Geometry: final body of the model. Coordinates: model frame, mm. A direction names the side the tool comes from. Coordinates: 2 decimals unless noted, no trailing zeros. Order: outer loops, then holes, each group sorted by start corner. A loop starts at its lowest first (then second) coordinate and runs counter-clockwise, first axis right, second up. Notation, with made-up numbers: M -17,70 L 40,70 A26 ccw 40,106 Z; hole C 59,-6.75 d6. An arc over 180 degrees is marked long. Write item = value, one per line.
from build123d import *

# Parameters (mm, degrees)
EXTRUDE_START       = 24.2
EXTRUDE_1_DEPTH     = 6
SKETCH_5_W          = 40
SKETCH_5_H          = 34
SKETCH_5_R          = 2
EXTRUDE_2_DEPTH     = 7
EXTRUDE_START_2     = -9.8
SKETCH_7_R          = 4.1
EXTRUDE_3_DEPTH     = 7
EXTRUDE_START_3     = -53
SKETCH_9_R          = 1.65
EXTRUDE_4_DEPTH     = 6
EXTRUDE_START_4     = -22.5
EXTRUDE_5_DEPTH     = 7
EXTRUDE_START_5     = 28
SKETCH_14_R         = 1.65
EXTRUDE_8_DEPTH     = 7
SKETCH_15_W         = 8
SKETCH_15_H         = 7
EXTRUDE_9_DEPTH     = 7
SKETCH_17_R         = 3
SKETCH_17_R_2       = 1.5
EXTRUDE_11_DEPTH    = 0.5
SKETCH_18_W         = 50.26694464
SKETCH_18_H         = 22.871129036
CUT_EXTRUDE_1_DEPTH = 50
SKETCH_19_W         = 15
SKETCH_19_H         = 30
SKETCH_19_R         = 1.75
SKETCH_19_W_2       = 30
SKETCH_19_H_2       = 15
EXTRUDE_12_DEPTH    = 7


with BuildPart() as part:
    # Sketch 4 → Extrude 1 (new body)
    with BuildSketch(Plane(origin=(0, 0, 0), x_dir=(1, 0, 0), z_dir=(0, 1, 0)).offset(EXTRUDE_START)):
        Polygon((-21, 22.5), (-28, 22.5), (-28, 29.5), (28, 29.5), (28, 22.5), (21, 22.5), align=None)
    extrude(amount=EXTRUDE_1_DEPTH)

    # Sketch 5 → Extrude 2 (add)
    with BuildSketch(Plane(origin=(0, 0, -29.5), x_dir=(-1, 0, 0), z_dir=(0, 0, -1))):
        with Locations((0, 7.2)):
            Rectangle(SKETCH_5_W, SKETCH_5_H)
        with Locations((-10, 21.7)):
            Circle(SKETCH_5_R, mode=Mode.SUBTRACT)
        with Locations(Location((10, 21.7, 0), (0, 0, 180))):
            Circle(SKETCH_5_R, mode=Mode.SUBTRACT)
        with Locations((10, 6.7)):
            Circle(SKETCH_5_R, mode=Mode.SUBTRACT)
        with Locations(Location((-10, 6.7, 0), (0, 0, 180))):
            Circle(SKETCH_5_R, mode=Mode.SUBTRACT)
    extrude(amount=-EXTRUDE_2_DEPTH)

    # Sketch 7 → Extrude 3 (add)
    with BuildSketch(Plane(origin=(0, 0, 0), x_dir=(1, 0, 0), z_dir=(0, 1, 0)).offset(EXTRUDE_START_2)):
        with BuildLine():
            Line((20, 22.5), (-20, 22.5))
            Line((-20, 22.5), (-20, 2.5))
            ThreePointArc((-20, 2.5), (-19.121320344, 0.378679656), (-17, -0.5))
            Line((-17, -0.5), (17, -0.5))
            ThreePointArc((17, -0.5), (19.121320344, 0.378679656), (20, 2.5))
            Line((20, 2.5), (20, 22.5))
        make_face()
        with Locations(Location((10, 10, 0), (0, 0, 90))):
            Circle(SKETCH_7_R, mode=Mode.SUBTRACT)
    extrude(amount=EXTRUDE_3_DEPTH)



with BuildPart() as body_2:
    # Sketch 9 → Extrude 4 (new body)
    with BuildSketch(Plane(origin=(22, 25.2, -43.868265324), x_dir=(0, 0, 1), z_dir=(1, 0, 0)).offset(EXTRUDE_START_3)):
        with BuildLine():
            Line((-8.631734676, 2.5), (21.368265324, 2.5))
            Line((21.368265324, 2.5), (21.368265324, 17.5))
            Line((21.368265324, 17.5), (-8.631734676, 17.5))
            ThreePointArc((-8.631734676, 17.5), (-16.131734676, 10), (-8.631734676, 2.5))
        make_face()
        with Locations(Location((-8.631734676, 10, 0), (0, 0, 270))):
            Circle(SKETCH_9_R, mode=Mode.SUBTRACT)
    extrude(amount=-EXTRUDE_4_DEPTH)


with BuildPart() as part_1:
    add(part.part)

    add(body_2.part)  # Extrude 5 merges body 2
    # Sketch 10 → Extrude 5 (add)
    with BuildSketch(Plane.XY.offset(EXTRUDE_START_4)):
        with BuildLine():
            Line((-31, 30.2), (-20, 30.2))
            Line((-20, 30.2), (-20, -9.8))
            Line((-20, -9.8), (-27, -9.8))
            ThreePointArc((-27, -9.8), (-29.828427125, -8.628427125), (-31, -5.8))
            Line((-31, -5.8), (-31, 30.2))
        make_face()
    extrude(amount=-EXTRUDE_5_DEPTH)

    # Sketch 14 → Extrude 8 (add)
    with BuildSketch(Plane(origin=(0, 0, 0), x_dir=(0, 0, -1), z_dir=(1, 0, 0)).offset(EXTRUDE_START_5)):
        with BuildLine():
            Line((22.5, 30.2), (32.5, 30.2))
            ThreePointArc((32.5, 30.2), (35.328427125, 29.028427125), (36.5, 26.2))
            Line((36.5, 26.2), (36.5, -5.8))
            ThreePointArc((36.5, -5.8), (35.328427125, -8.628427125), (32.5, -9.8))
            Line((32.5, -9.8), (22.5, -9.8))
            Line((22.5, -9.8), (22.5, 30.2))
        make_face()
        with Locations((28.5, 15.2)):
            Circle(SKETCH_14_R, mode=Mode.SUBTRACT)
        with Locations((32.5, 15.2)):
            Circle(SKETCH_14_R, mode=Mode.SUBTRACT)
    extrude(amount=EXTRUDE_8_DEPTH)

    # Sketch 15 → Extrude 9 (add)
    with BuildSketch(Plane(origin=(0, 0, 0), x_dir=(1, 0, 0), z_dir=(0, 1, 0)).offset(EXTRUDE_START_2)):
        with Locations((24, 26)):
            Rectangle(SKETCH_15_W, SKETCH_15_H)
    extrude(amount=EXTRUDE_9_DEPTH)

    # Sketch 17 → Extrude 11 (add)
    with BuildSketch(Plane(origin=(-31, 0, 0), x_dir=(0, 0, -1), z_dir=(1, 0, 0))):
        with Locations(Location((52.5, 15.2, 0), (0, 0, 90))):
            Circle(SKETCH_17_R)
        with Locations(Location((52.5, 15.2, 0), (0, 0, 90))):
            Circle(SKETCH_17_R_2, mode=Mode.SUBTRACT)
    extrude(amount=EXTRUDE_11_DEPTH)

    # Sketch 18 → Cut-Extrude 1 (cut)
    with BuildSketch(Plane.XY.offset(-22.5)):
        Rectangle(SKETCH_18_W, SKETCH_18_H)
    extrude(amount=CUT_EXTRUDE_1_DEPTH, mode=Mode.SUBTRACT)

    # Sketch 19 → Extrude 12 (add)
    # profile 1 of 4: a face of its own
    with BuildSketch(Plane.XY.offset(EXTRUDE_START_4)):
        with Locations((0, 45.2)):
            Rectangle(SKETCH_19_W, SKETCH_19_H)
        with Locations((0, 53.2)):
            Circle(SKETCH_19_R, mode=Mode.SUBTRACT)
    # profile 2 of 4: a face of its own
    with BuildSketch(Plane.XY.offset(EXTRUDE_START_4)):
        with Locations((-52, 15.2)):
            Rectangle(SKETCH_19_W_2, SKETCH_19_H_2)
        with Locations((-60, 15.2)):
            Circle(SKETCH_19_R, mode=Mode.SUBTRACT)
    # profile 3 of 4: a face of its own
    with BuildSketch(Plane.XY.offset(EXTRUDE_START_4)):
        with Locations((50, 2.7)):
            Rectangle(SKETCH_19_W_2, SKETCH_19_H_2)
        with Locations((58, 2.7)):
            Circle(SKETCH_19_R, mode=Mode.SUBTRACT)
    # profile 4 of 4: a face of its own
    with BuildSketch(Plane.XY.offset(EXTRUDE_START_4)):
        with Locations((0, -24.8)):
            Rectangle(SKETCH_19_W, SKETCH_19_H)
        with Locations((0, -32.8)):
            Circle(SKETCH_19_R, mode=Mode.SUBTRACT)
    extrude(amount=-EXTRUDE_12_DEPTH)


solid = part_1.part
1) Mould query, pull axis Y, two halves, no side actions, for faces 1 (the face through (20, 11, -26)), 2 (the face through (21, 30.2, -26)), 3 (the face through (7.5, 45, -26)). Classes: pulls with the +Y half, pulls with the -Y half, needs draft (parallel to the pull), parting line crosses it, or undercut.
Numbers:
face_1 = undercut
face_2 = pulls with the +Y half
face_3 = needs draft
2) Section B-B, the plane y = 53.2. Return loops of the section in (x, z), and give its area (3 significant figures).
Numbers:
outline = M -7.5,-29.5 L -1.75,-29.5 L -1.75,-22.5 L -7.5,-22.5 Z; M 1.75,-29.5 L 7.5,-29.5 L 7.5,-22.5 L 1.75,-22.5 Z
area = 80.5 mm²
3) Section C-C, the plane z = -46. Return loops of the section in (x, y), and give its area (3 significant figures).
Numbers:
outline = M -37,7.7 L -31,7.7 L -31,22.7 L -37,22.7 Z
area = 90.0 mm²
4) Line query: L1, parallel to Y at x = 10, z = -25; L2, parallel to Y at x = 58, z = -27.25; L3, parallel to Y at x = 20.5, z = -24. Output: solid intervals per line, ascending.
Numbers:
L1 = -9.8 to 4.7, 8.7 to 19.7, 23.7 to 30.2
L2 = -4.8 to 0.95, 4.45 to 10.2
L3 = -9.8 to -2.8, 24.2 to 30.2
5) Pin query (flat end, axial travel): pin 1 (5.5 mm diameter, centred on y = 48, z = -27.5, fed in from -X); pin 2 (5.5 mm diameter, centred on y = 2.5, z = -26, fed in from -X); pin 3 (2.5 mm diameter, centred on x = 10, y = 21.7, fed in from -Z); pin 4 (3.5 mm diameter, centred on x = 44, z = -26, fed in from +Y). Return the tip coordinate at first contact, or that it passes through.
Numbers:
pin_1 = -7.5
pin_2 = -31
pin_3 = through
pin_4 = 10.2
6) Section D-D, the plane x = 41.5. Return loops of the section in (y, z).
Numbers:
outline = M -4.8,-29.5 L 10.2,-29.5 L 10.2,-22.5 L -4.8,-22.5 Z
7) Section A-A, the plane x = 0. Return loops of the section in (y, z), and give its area (3 significant figures).
Numbers:
outline = M -39.8,-29.5 L -34.55,-29.5 L -34.55,-22.5 L -39.8,-22.5 Z; M -31.05,-29.5 L 51.45,-29.5 L 51.45,-22.5 L -31.05,-22.5 Z; M 54.95,-29.5 L 60.2,-29.5 L 60.2,-22.5 L 54.95,-22.5 Z
area = 651 mm²
8) Set-up query: faces 4 (the face through (-19, 30.2, -26)), 5 (the face through (31.45, 14.2, -27.19)), 6 (the face through (-17, -9.8, -26)), 7 (the face through (50, -4.8, -26)). Return all of +Z, -Z, +X, -X, +Y, -Y with unobstructed straight access to the full face (end or side cutting, diameter ignored); none if empty.
Numbers:
face_4 = +Z, -Z, -X, +Y
face_5 = +X
face_6 = +Z, -Z, -X, -Y
face_7 = +Z, -Z, +X, -Y
